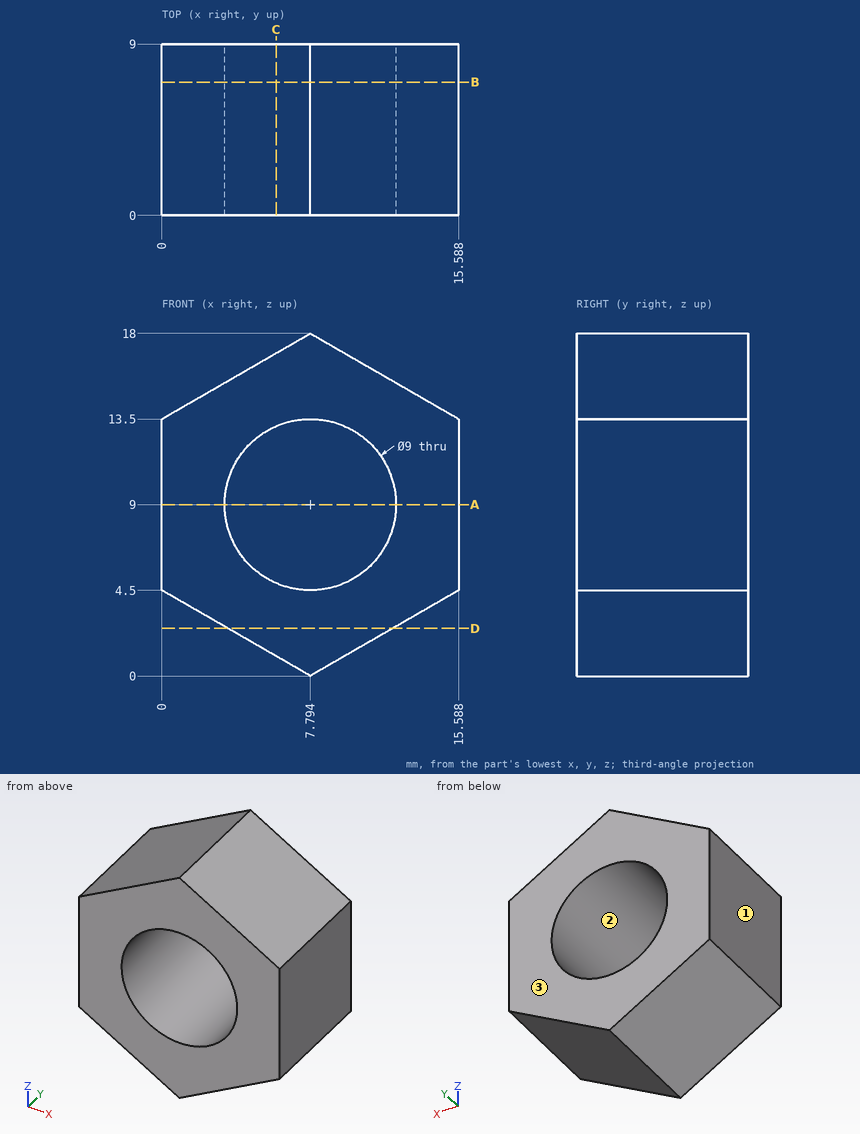
Job drawing, mm, ordinate dimensions from the low corner. One solid piece. Coordinates: 2 decimals unless noted, no trailing zeros. Loops run counter-clockwise (first coordinate to the right, second up) from the corner with the lowest first, then second, coordinate; pieces in that order, holes last. Notation, with made-up numbers: (1, -30) - (60, -30) arc R16 cw to (60, 1) - close; hole circle Ø3 at (54.25, 61.5). An arc over 180 degrees is marked (long way). Write item = value, one per line. Start each with the question number.
Q1. Cut at B-B, the plane y = 7. List the corners of the cut face in (x, z) (1 decimal), then the cut area to 3 significant figures.
Q2. Cut at C-C, the plane x = 6. List the corners of the cut face in (y, z) (1 decimal).
Q3. Flat gauge pins, fed straight in: pin 1 Ø3 at (x, y) = (5, 5) entering from -Z; pin 2 Ø8 at (x, z) = (9, 3) entering from -Y; pin 3 Ø1.5 at (x, y) = (13.5, 1) entering from +Z; pin 4 Ø2 at (y, z) = (5.5, 15) entering from -X (1 decimal). Where does each tip first touch, or does it go through?
Q4. Drill centre lines: L1, parallel to X at y = 5.5, z = 9 (1 decimal); L2, parallel to Z at x = 7.25, y = 5 (1 decimal); L3, parallel to X at y = 6.25, z = 8.25. Where is each one in solid material? Low to high.
Q5. Cut at D-D, the plane z = 2.5. List the corners of the cut face in (x, y) (1 decimal).
Q6. Cut at A-A, the plane z = 9. List the corners of the cut face in (x, y) (1 decimal).
Q7. Pull direction X, two halves, no side cores. Call the marked faces 1, 2 and 3: pulls with the +X half, pulls with the -X half, needs draft (parallel to the pull), parting line crosses it, or undercut.
Computed:
q1.outline = (0, 4.5) - (7.8, 0) - (15.6, 4.5) - (15.6, 13.5) - (7.8, 18) - (0, 13.5) - close; hole circle Ø9 at (7.8, 9)
q1.area = 147 mm²
q2.outline = (0, 1) - (9, 1) - (9, 4.9) - (0, 4.9) - close; (0, 13.1) - (9, 13.1) - (9, 17) - (0, 17) - close
q3.pin_1 = 0.75
q3.pin_2 = 0
q3.pin_3 = 15.14
q3.pin_4 = 0.9
q4.L1 = 0 to 3.3, 12.3 to 15.6
q4.L2 = 0.3 to 4.5, 13.5 to 17.7
q4.L3 = 0 to 3.36, 12.23 to 15.59
q5.outline = (3.5, 0) - (12.1, 0) - (12.1, 9) - (3.5, 9) - close
q6.outline = (0, 0) - (3.3, 0) - (3.3, 9) - (0, 9) - close; (12.3, 0) - (15.6, 0) - (15.6, 9) - (12.3, 9) - close
q7.face_1 = pulls with the -X half
q7.face_2 = undercut
q7.face_3 = needs draft
